```python
from build123d import *

# Parameters (mm, degrees)
CYLINDER_R        = 9
CYLINDER_DEPTH    = 1.2
CYLINDER001_R     = 8
CYLINDER001_DEPTH = 75
CYLINDER002_R     = 4
CYLINDER002_DEPTH = 76.2
CYLINDER003_R     = 6.8
CYLINDER003_DEPTH = 75
FILLET_R          = 0.3


with BuildPart() as part:
    # Cylinder → Cylinder (join)
    with BuildSketch(Plane.XY):
        Circle(CYLINDER_R)
    extrude(amount=CYLINDER_DEPTH)

    # Cylinder001 → Cylinder001 (join)
    with BuildSketch(Plane.XY.offset(1.2)):
        Circle(CYLINDER001_R)
    extrude(amount=CYLINDER001_DEPTH)

    # Cylinder002 → Cylinder002 (cut)
    with BuildSketch(Plane.XY):
        Circle(CYLINDER002_R)
    extrude(amount=CYLINDER002_DEPTH, mode=Mode.SUBTRACT)

    # Cylinder003 → Cylinder003 (cut)
    with BuildSketch(Plane.XY.offset(1.2)):
        Circle(CYLINDER003_R)
    extrude(amount=CYLINDER003_DEPTH, mode=Mode.SUBTRACT)

    # Fillet
    fillet_edges = [part.edges().sort_by_distance(p)[0] for p in [
        (-9, 0, 1.2),
        (-8, 0, 76.2),
        (-6.8, 0, 76.2),
    ]]
    fillet(fillet_edges, radius=FILLET_R)


solid = part.part
```
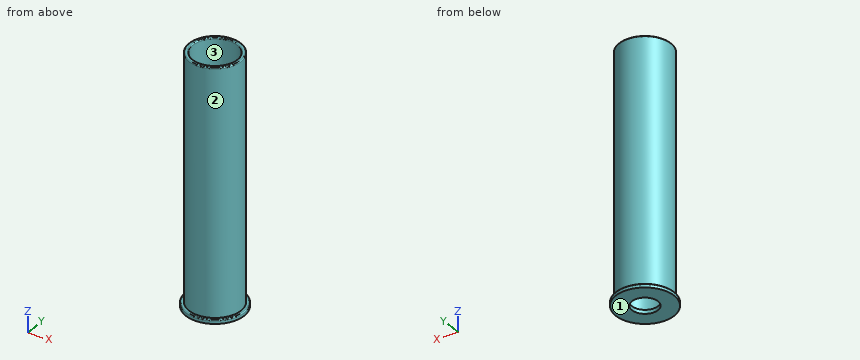
The listing builds one solid part. Answer for the finished solid, in the listing's coordinates (mm). Face numbers are marked on the shaded views. Round coordinates to 2 decimals unless told otherwise and drop trailing zeros. Loops run counter-clockwise (first coordinate to the right, second up) from the corner with the lowest first, then second, coordinate; pieces in that order, holes last. Notation, with made-up numbers: (49.25, -16) - (102.25, -16) arc R32 ccw to (102.25, 19) - close; hole circle Ø4 at (75, 32). An arc over 180 degrees is marked (long way). Use one line per item in the form item = value. Start each with the question number.
1. For a pull along Y with two mould halves and no side action, classify the marked faces 1, 2 and 3 as pulls with the +Y half, pulls with the -Y half, needs draft (parallel to the pull), parting line crosses it, or undercut.
2. The part is cut by section C-C on z = 56.5. Determine the outline of the cut face in (x, y), then the cut area to 3 significant figures.
3. Given pin 1 Ø10.5 at (x, y) = (0, 0) entering from +Z; pin 2 Ø4 at (x, z) = (-6.5, 50) entering from -Y; pin 3 Ø4 at (y, z) = (-7, 40.5) entering from -X (3 decimals), each flat-ended and moving along its own axis, determine where each tip first touches the part or whether it passes through.
4. Consider line 1 (Y direction, x = 0, z = 23); line 2 (Y direction, x = 0, z = 0.85); line 3 (Z direction, x = 3.75, y = -4.5). Determine where each line is inside the solid, lowest interval first. Write a range as [from, to].
5. The part is cut by section A-A on x = 0. Determine the outline of the cut face in (y, z).
Geometry check:
q1.face_1 = needs draft
q1.face_2 = parting line crosses it
q1.face_3 = undercut
q2.outline = circle Ø16 at (0, 0); hole circle Ø13.6 at (0, 0)
q2.area = 55.8 mm^2
q3.pin_1 = 1.2
q3.pin_2 = -6.61
q3.pin_3 = -6.245
q4.line_1 = [-8, -6.8], [6.8, 8]
q4.line_2 = [-9, -4], [4, 9]
q4.line_3 = [0, 1.2]
q5.outline = (-9, 0) - (-4, 0) - (-4, 1.2) - (-6.8, 1.2) - (-6.8, 75.9) arc R0.3 ccw to (-7.1, 76.2) - (-7.7, 76.2) arc R0.3 ccw to (-8, 75.9) - (-8, 1.2) - (-8.7, 1.2) arc R0.3 ccw to (-9, 0.9) - close; (4, 0) - (9, 0) - (9, 0.9) arc R0.3 ccw to (8.7, 1.2) - (8, 1.2) - (8, 75.9) arc R0.3 ccw to (7.7, 76.2) - (7.1, 76.2) arc R0.3 ccw to (6.8, 75.9) - (6.8, 1.2) - (4, 1.2) - close
